```python
from build123d import *

# Parameters (mm, degrees)
F0_R     = 2.25
F1_DEPTH = 5
F2_W     = 22.901535
F2_H     = 5
F3_DEPTH = 30


with BuildPart() as f1:
    # F0 (on Right) → F1 (new body)
    with BuildSketch(Plane.YZ):
        Polygon((62, 70.5), (-68, 70.5), (-68, -85.5), (-68, -107.009701), (-45.098465, -107.009701), (-45.098465, -85.5), (39.098465, -85.5), (39.098465, -107.009701), (62, -107.009701), (62, -85.5), align=None)
        with Locations((-10, -55.8)):
            Circle(F0_R, mode=Mode.SUBTRACT)
        with Locations((10, -55.8)):
            Circle(F0_R, mode=Mode.SUBTRACT)
        with Locations((-10, 55.53)):
            Circle(F0_R, mode=Mode.SUBTRACT)
        with Locations((10, 55.53)):
            Circle(F0_R, mode=Mode.SUBTRACT)
    extrude(amount=F1_DEPTH)

    # F2 (on face) → F3 (join)
    with BuildSketch(Plane.YZ.offset(5)):
        with Locations((-56.549233, -104.509701)):
            Rectangle(F2_W, F2_H)
        with Locations((50.549233, -104.509701)):
            Rectangle(F2_W, F2_H)
    extrude(amount=F3_DEPTH)


solid = f1.part
```
CAD build for the part. Positions are in the model's coordinates, mm. A direction names the side the tool comes from. Round coordinates to 2 decimals unless told otherwise and drop trailing zeros. Loops run counter-clockwise (first coordinate to the right, second up) from the corner with the lowest first, then second, coordinate; pieces in that order, holes last. Notation, with made-up numbers: M 51.25,56 L 101.25,56 A28 ccw 101.25,94 Z; hole C 19,-17.75 d1. An arc over 180 degrees is marked long. Return JSON: item names as keys, results as strings. Group by question number.
(1) Saw through at C-C, the plane z = -55.8. List the corners of the cut face in (x, y), and give its area (3 significant figures).
(2) Mould opens along Z. For faces 6 (the flat face through (17, 50, -107.01)), 7 (the cylindrical face through (2.46, -10.29, -53.57)), 8 (the flat face through (2, -2, 70.5)), 9 (the cylindrical face through (2.46, 9.71, 57.76)) say: +Z half, -Z half, draft (parallel to the pull), parting line (faces both ways), or undercut.
(3) Wall check: probe 1 along Z at (x, y) = (2, -10); probe 2 along Z at (x, y) = (20, 42); probe 3 along X at (y, z) = (-53.5, -18.5). Give the ranges that are in metal, low to high. Write a range as [from, to].
(4) Saw through at D-D, the plane y = 45.5. List the corners of the cut face in (x, z).
(5) Saw through at A-A, the plane y = 10. List the corners of the cut face in (x, z).
(6) Drop flat-ended pins along their axis: P1, Ø2.5, axis at y = 10, z = -55.8, coming from the +X side; P2, Ø7, axis at x = 20.5, y = -54, coming from the +Z side; P3, Ø1.5, axis at x = 1.5, y = -19.5, coming from the -Z side; P4, Ø5, axis at y = -10, z = 55.53, coming from the +X side. Give the stop position or say it passes through.
(7) Tool access for faces 1 (the flat face through (35, -57, -104)), 2 (the flat face through (2, -68, -17)), 3 (the flat face through (20, 50, -102.01)), 4 (the flat face through (20, -45.098, -105)), 5 (the flat face through (2, -4, -85.5)): list every direction of +Z, -Z, +X, -X, +Y, -Y with a clear straight run to the whole face (end or side of a thin tool).
(8) Saw through at B-B, the plane x = 20.5. List the corners of the cut face in (y, z), and give its area (3 significant figures).
Answer list:
{
 "1": {"outline": "M 0,-68 L 5,-68 L 5,-12.25 L 0,-12.25 Z; M 0,-7.75 L 5,-7.75 L 5,7.75 L 0,7.75 Z; M 0,12.25 L 5,12.25 L 5,62 L 0,62 Z", "area": "605 mm2"},
 "2": {"face 6": "-Z half", "face 7": "undercut", "face 8": "+Z half", "face 9": "undercut"},
 "3": {"probe 1": "[-85.5, -58.05], [-53.55, 53.28], [57.78, 70.5]", "probe 2": "[-107.01, -102.01]", "probe 3": "[0, 5]"},
 "4": {"outline": "M 0,-107.01 L 35,-107.01 L 35,-102.01 L 5,-102.01 L 5,70.5 L 0,70.5 Z"},
 "5": {"outline": "M 0,-85.5 L 5,-85.5 L 5,-58.05 L 0,-58.05 Z; M 0,-53.55 L 5,-53.55 L 5,53.28 L 0,53.28 Z; M 0,57.78 L 5,57.78 L 5,70.5 L 0,70.5 Z"},
 "6": {"P1": "through", "P2": "z = -102.01", "P3": "z = -85.5", "P4": "x = 5"},
 "7": {"face 1": "+Z, -Z, +X, +Y, -Y", "face 2": "+Z, -Z, +X, -X, -Y", "face 3": "+Z, +X, +Y, -Y", "face 4": "+Z, -Z, +X, -X", "face 5": "-Z, +X, -X"},
 "8": {"outline": "M -68,-107.01 L -45.1,-107.01 L -45.1,-102.01 L -68,-102.01 Z; M 39.1,-107.01 L 62,-107.01 L 62,-102.01 L 39.1,-102.01 Z", "area": "229 mm2"}
}
